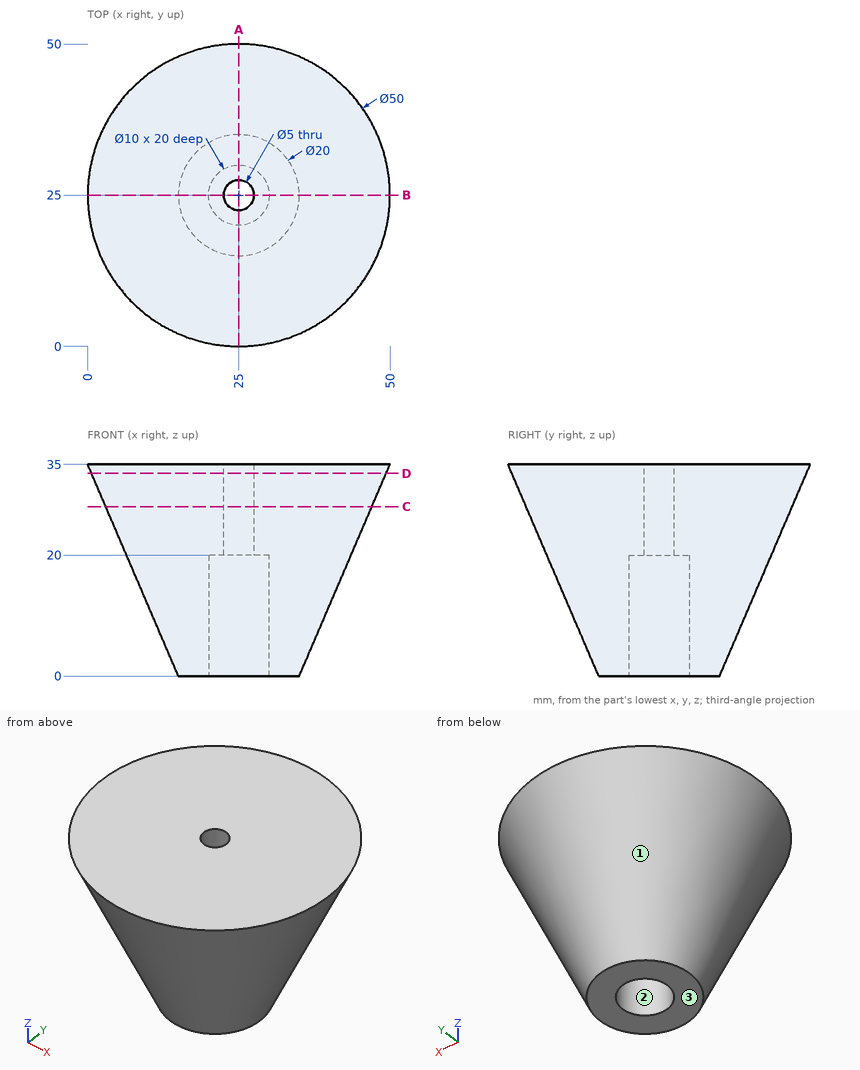
Verification items for this drawing (mm, ordinates from the low corner). Coordinates: 2 decimals unless noted, no trailing zeros. Loops run counter-clockwise (first coordinate to the right, second up) from the corner with the lowest first, then second, coordinate; pieces in that order, holes last. Notation, with made-up numbers: (22.5, 14.25) -> (58.5, 14.25) arc R37 ccw to (58.5, 53.25) -> close; hole circle Ø10 at (67, 20). An arc over 180 degrees is marked (long way). Put each result on its own line as item: value.
1. Section check A-A, the plane x = 25. Record the boundary of the cut face in (y, z), then the cut area to 3 significant figures.
Result set:
outline: (0, 35) -> (15, 0) -> (20, 0) -> (20, 20) -> (22.5, 20) -> (22.5, 35) -> close; (27.5, 20) -> (30, 20) -> (30, 0) -> (35, 0) -> (50, 35) -> (27.5, 35) -> close
area: 950 mm^2
2. Section check C-C, the plane z = 28. Record the boundary of the cut face in (x, y).
Result set:
outline: circle Ø44 at (25, 25); hole circle Ø5 at (25, 25)
3. Gauge pin test, flat ends, axial feed: P1, Ø1.5, axis at x = 25, y = 44, coming from the -Z side; P2, Ø12, axis at x = 24.5, z = 7.5, coming from the -Y side; P3, Ø12, axis at x = 16.5, z = 6, coming from the -Y side. Record the tip position at first contact, or that the pin passes through.
Result set:
P1: stops at z = 19.25
P2: stops at y = 9.22
P3: stops at y = 11.22
4. Section check D-D, the plane z = 33.5. Record the boundary of the cut face in (x, y), then the cut area to 3 significant figures.
Result set:
outline: circle Ø48.71 at (25, 25); hole circle Ø5 at (25, 25)
area: 1,840 mm^2
5. Thickness scan on line 1 (X direction, y = 26.5, z = 15.5); line 2 (Y direction, x = 25, z = 24); line 3 (X direction, y = 25, z = 29). Record the ranges inside material, lowest first.
Result set:
line 1: x = 8.42 to 20.23, 29.77 to 41.58
line 2: y = 4.71 to 22.5, 27.5 to 45.29
line 3: x = 2.57 to 22.5, 27.5 to 47.43
6. Mould release check, pull along X, two halves, no side actions. Record for the marked faces 1, 2 and 3: pulls with the +X half, pulls with the -X half, needs draft (parallel to the pull), parting line crosses it, or undercut.
Result set:
face 1: parting line crosses it
face 2: undercut
face 3: needs draft
